For this review, use the dimensioned drawing (mm, ordinates from the lowest corner) and the shaded views. A direction names the side the tool comes from. Coordinates: 2 decimals unless noted, no trailing zeros. Loops run counter-clockwise (first coordinate to the right, second up) from the corner with the lowest first, then second, coordinate; pieces in that order, holes last. Notation, with made-up numbers: (72, 26.25) - (111, 26.25) arc R29 ccw to (111, 58.25) - close; hole circle Ø1 at (71.5, 52). An arc over 180 degrees is marked (long way). Use one line per item in the form item = value. Start each with the question number.
(1) Add section C-C (x = 8.25). State the section outline as (y, z) points.
(2) Add section A-A (x = 1.5). State the section outline as (y, z) points.
(3) For L1, parallel to X at y = 0.3, z = 4; L2, parallel to X at y = 20.5, z = 2, list the stretches that pass through material, from the lowest coordinate up.
(4) Add section D-D (y = 14.5). State the section outline as (x, z) points, plus the area to 3 significant figures.
(5) Add section B-B (z = 4). Count the separate pieces of the cut face and the enclosed holes in it.
(6) Tool access review of the marked faces 1 and 2: name each direction out of +Z, -Z, +X, -X, +Y, -Y from which nothing blocks a thin tool from reaching the whole face with its end or side.
(7) Clearance check with flat-ended pins moving along their axes: pin 1 Ø4.5 at (x, z) = (18, 4) entering from +Y; pin 2 Ø4 at (y, z) = (9, 4) entering from +X; pin 3 Ø1.5 at (y, z) = (3, 5.5) entering from +X; pin 4 Ø3 at (x, z) = (9, 4) entering from +Y. State where each tip first meets the part, or that it passes through.
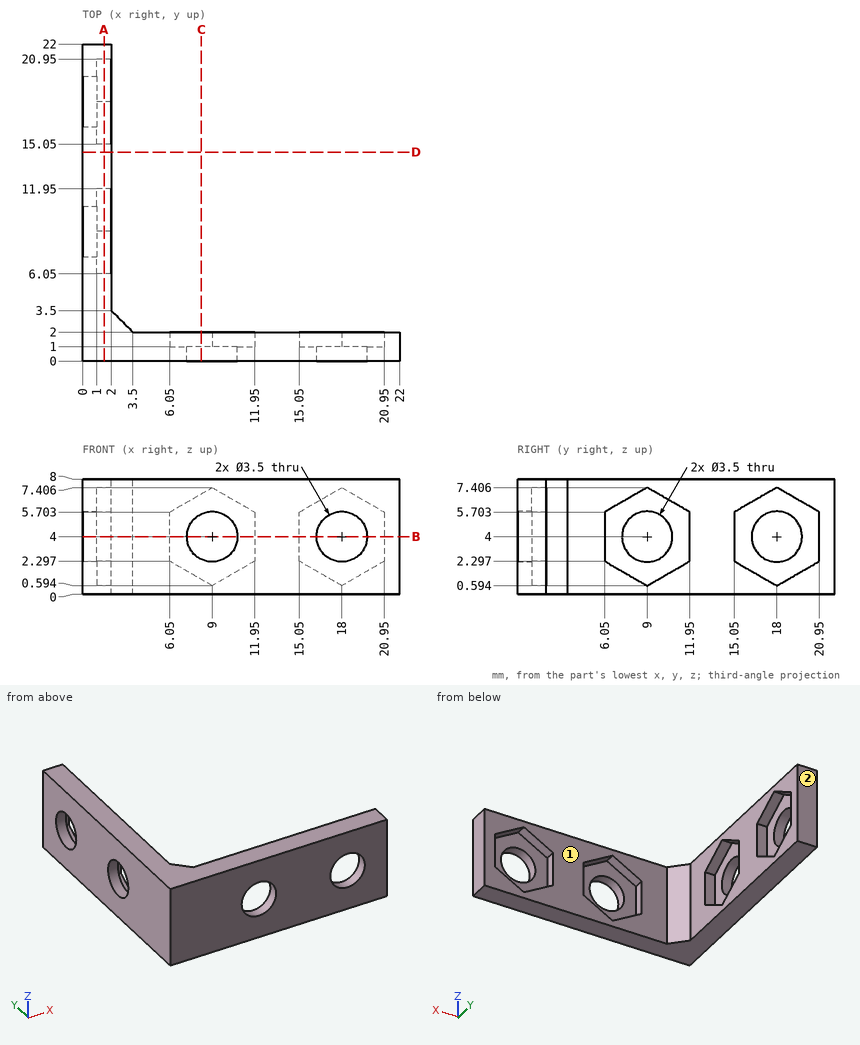
Computed values:
q1.outline = (0, 0) - (2, 0) - (2, 1.03) - (1, 1.03) - (1, 2.42) - (0, 2.42) - close; (0, 5.58) - (1, 5.58) - (1, 6.97) - (2, 6.97) - (2, 8) - (0, 8) - close
q2.outline = (0, 0) - (22, 0) - (22, 8) - (0, 8) - close; hole (6.05, 2.3) - (9, 0.59) - (11.95, 2.3) - (11.95, 5.7) - (9, 7.41) - (6.05, 5.7) - close; hole (15.05, 2.3) - (18, 0.59) - (20.95, 2.3) - (20.95, 5.7) - (18, 7.41) - (15.05, 5.7) - close
q3.L1 = 0 to 7.25, 10.75 to 16.25, 19.75 to 22
q3.L2 = 0 to 2
q4.outline = (0, 0) - (2, 0) - (2, 8) - (0, 8) - close
q4.area = 16.0 mm^2
q5.separate_pieces = 5
q5.enclosed_holes = 0
q6.face_1 = +Z, -Z, +X, +Y
q6.face_2 = +Z, -Z, +X, -X, +Y
q7.pin_1 = 1
q7.pin_2 = 1
q7.pin_3 = 3.25
q7.pin_4 = through
